Read the model definition and answer for the solid it produces. Units are mm, in the model's axes. A direction names the side the tool comes from. Coordinates: 2 decimals unless noted, no trailing zeros. Write each loop counter-clockwise with the first axis right and the second up, starting at its lowest first coordinate (ties: lowest second). Pieces come first, ordered by that corner, then holes. Notation, with made-up numbers: (-14, 63) -> (-5, 63) arc R30 cw to (-5, 87) -> close; hole circle Ø6 at (27, -34). An arc over 180 degrees is marked (long way). Use CSV: the item, a comma, the result in double quotes.
from build123d import *

# Parameters (mm, degrees)
ESBO_O1_R                = 1.5
RESSALTO_EXTRUS_O1_DEPTH = 2


with BuildPart() as part:
    # Esboço1 → Ressalto-extrusão1 (new body)
    with BuildSketch(Plane.XY):
        with BuildLine():
            Line((24.828910237, 4.947115543), (-67.47493734, 4.947115543))
            ThreePointArc((-67.47493734, 4.947115543), (-72.976635365, 4.201423413), (-68.533513234, 0.872248794))
            Line((-68.533513234, 0.872248794), (-39.094485287, -22.491099002))
            Line((-39.094485287, -22.491099002), (-39.094485287, -52.920988494))
            Line((-39.094485287, -52.920988494), (-50.165018851, -67.855248208))
            ThreePointArc((-50.165018851, -67.855248208), (-54.378358474, -71.627569421), (-48.752314099, -71.052884457))
            Line((-48.752314099, -71.052884457), (6.078910237, -71.052884457))
            ThreePointArc((6.078910237, -71.052884457), (11.761262781, -71.628269251), (7.481508074, -67.846219841))
            Line((7.481508074, -67.846219841), (-3.636404062, -52.83035158))
            Line((-3.636404062, -52.83035158), (-3.636404062, -22.558447224))
            Line((-3.636404062, -22.558447224), (25.887486132, 0.872248794))
            ThreePointArc((25.887486132, 0.872248794), (30.330608262, 4.201423413), (24.828910237, 4.947115543))
        make_face()
        with Locations((-51.658717817, -70.426041486)):
            Circle(ESBO_O1_R, mode=Mode.SUBTRACT)
        Polygon((-22.823013551, -36.008314403), (-22.823013551, -68.926041486), (-47.22441071, -68.926041486), align=None, mode=Mode.SUBTRACT)
        Polygon((-36.094485287, -24.871953544), (-24.892352245, -33.762169987), (-36.094485287, -48.873958703), align=None, mode=Mode.SUBTRACT)
        with Locations((9.012690715, -70.426041486)):
            Circle(ESBO_O1_R, mode=Mode.SUBTRACT)
        Polygon((-19.823013551, -36.010232621), (4.548209245, -68.926041486), (-19.823013551, -68.926041486), align=None, mode=Mode.SUBTRACT)
        Polygon((-21.323013551, -33.984330445), (-21.322839799, -33.984565114), (-21.323013551, -33.984799507), align=None, mode=Mode.SUBTRACT)
        Polygon((-6.636404062, -24.939301765), (-6.636404062, -48.778547228), (-17.754316199, -33.762678967), align=None, mode=Mode.SUBTRACT)
        Polygon((-42.445301093, -16.001887011), (-22.823013551, 0.011039778), (-22.823013551, -31.574491147), align=None, mode=Mode.SUBTRACT)
        with Locations((-70.073013551, 3.447115543)):
            Circle(ESBO_O1_R, mode=Mode.SUBTRACT)
        Polygon((-65.061973687, 1.947115543), (-25.195486483, 1.947115543), (-44.850847826, -14.092801389), align=None, mode=Mode.SUBTRACT)
        Polygon((-19.823013551, -31.574491147), (-19.823013551, 0.011063284), (-0.200409257, -16.00163563), align=None, mode=Mode.SUBTRACT)
        Polygon((2.205145312, -14.09254379), (-17.450497364, 1.947115543), (22.415946584, 1.947115543), align=None, mode=Mode.SUBTRACT)
        with Locations((27.426986449, 3.447115543)):
            Circle(ESBO_O1_R, mode=Mode.SUBTRACT)
    extrude(amount=RESSALTO_EXTRUS_O1_DEPTH)


solid = part.part
1. A cutting plane is placed at C-C (y = -37.5). Give the vertices of the cut face in (x, z).
Solutions:
outline,"(-39.09, 0) -> (-36.09, 0) -> (-36.09, 2) -> (-39.09, 2) -> close; (-27.66, 0) -> (-23.93, 0) -> (-23.93, 2) -> (-27.66, 2) -> close; (-22.82, 0) -> (-19.82, 0) -> (-19.82, 2) -> (-22.82, 2) -> close; (-18.72, 0) -> (-14.99, 0) -> (-14.99, 2) -> (-18.72, 2) -> close; (-6.64, 0) -> (-3.64, 0) -> (-3.64, 2) -> (-6.64, 2) -> close"
2. Find the intervals of material crossed by line 1 along X through (y, z) = (-67, 1.05); line 2 along Y through (x, z) = (-11.5, 1.4); line 3 along X through (y, z) = (-6, 0.25), in increasing order.
Solutions:
line 1,"x = -49.53 to -45.8, -22.82 to -19.82, 3.12 to 6.85"
line 2,"y = -71.05 to -68.93, -47.25 to -42.21, -28.8 to -24.97, -6.78 to -2.91, 1.95 to 4.95"
line 3,"x = -59.87 to -55.05, -34.93 to -30.19, -22.82 to -19.82, -12.46 to -7.71, 12.4 to 17.23"
3. A tool of negligible diameter and unlimited length cuts with its end or side. For faces 1 (the flat face through (-21, 4.947, 1)), 2 (the flat face through (-6.636, -37, 1)), from which of +Z, -Z, +X, -X, +Y, -Y can it reach the whole face along a straight path? Write none if from no direction.
Solutions:
face 1,"+Z, -Z, +Y"
face 2,"+Z, -Z"
4. A cutting plane is placed at A-A (x = 14). Give the vertices of the cut face in (y, z).
Solutions:
outline,"(-8.56, 0) -> (-4.73, 0) -> (-4.73, 2) -> (-8.56, 2) -> close; (1.95, 0) -> (4.95, 0) -> (4.95, 2) -> (1.95, 2) -> close"
5. A cutting plane is placed at B-B (x = -51.5). Give the vertices of the cut face in (y, z).
Solutions:
outline,"(-73.4, 0) -> (-71.92, 0) -> (-71.92, 2) -> (-73.4, 2) -> close; (-68.93, 0) -> (-67.46, 0) -> (-67.46, 2) -> (-68.93, 2) -> close; (-12.65, 0) -> (-8.82, 0) -> (-8.82, 2) -> (-12.65, 2) -> close; (1.95, 0) -> (4.95, 0) -> (4.95, 2) -> (1.95, 2) -> close"
6. Each of these flat-tipped pins is pushed along its axis until it touches: pin 1 Ø4 at (x, y) = (27.43, 3.45) entering from +Z; pin 2 Ø1 at (y, z) = (-36, 1) entering from -X; pin 3 Ø1 at (x, z) = (-12.5, 1) entering from -Y; pin 4 Ø0.6 at (x, z) = (11, 1.5) entering from -Y. Where does it stop, or does it pass through?
Solutions:
pin 1,"stops at z = 2"
pin 2,"stops at x = -39.09"
pin 3,"stops at y = -71.05"
pin 4,"stops at y = -72.91"
7. A cutting plane is placed at D-D (y = -19). Give the vertices of the cut face in (x, z).
Solutions:
outline,"(-43.49, 0) -> (-38.67, 0) -> (-38.67, 2) -> (-43.49, 2) -> close; (-22.82, 0) -> (-19.82, 0) -> (-19.82, 2) -> (-22.82, 2) -> close; (-3.98, 0) -> (0.85, 0) -> (0.85, 2) -> (-3.98, 2) -> close"
